```python
from build123d import *

# Parameters (mm, degrees)
SKETCH2_W           = 130
SKETCH2_H           = 70
BOSS_EXTRUDE1_DEPTH = 100
SKETCH3_W           = 104
SKETCH3_H           = 74
CUT_EXTRUDE1_DEPTH  = 67
SKETCH4_W           = 10
SKETCH4_H           = 10
CUT_EXTRUDE2_DEPTH  = 55
SKETCH5_W           = 104
SKETCH5_H           = 10
CUT_EXTRUDE3_DEPTH  = 67
SKETCH6_W           = 10
SKETCH6_H           = 74
CUT_EXTRUDE4_DEPTH  = 67
SKETCH9_R           = 1.75
CUT_EXTRUDE5_DEPTH  = 67
SKETCH10_R          = 4
CUT_EXTRUDE6_DEPTH  = 5
SKETCH12_R          = 4
CUT_EXTRUDE7_DEPTH  = 5
SKETCH13_R          = 4
CUT_EXTRUDE8_DEPTH  = 5
SKETCH14_R          = 4
CUT_EXTRUDE9_DEPTH  = 5
SKETCH15_W          = 3
SKETCH15_H          = 3
BOSS_EXTRUDE2_DEPTH = 5


with BuildPart() as part:
    # Sketch2 → Boss-Extrude1 (new body)
    with BuildSketch(Plane(origin=(0, 0, 0), x_dir=(1, 0, 0), z_dir=(0, 1, 0))):
        with Locations((65, 35)):
            Rectangle(SKETCH2_W, SKETCH2_H)
    extrude(amount=BOSS_EXTRUDE1_DEPTH)

    # Sketch3 → Cut-Extrude1 (cut)
    with BuildSketch(Plane(origin=(0, 0, -70), x_dir=(-1, 0, 0), z_dir=(0, 0, -1))):
        with Locations((-65, 50)):
            Rectangle(SKETCH3_W, SKETCH3_H)
    extrude(amount=-CUT_EXTRUDE1_DEPTH, mode=Mode.SUBTRACT)

    # Sketch4 → Cut-Extrude2 (cut)
    with BuildSketch(Plane.XY):
        with Locations((5, 95)):
            Rectangle(SKETCH4_W, SKETCH4_H)
        with Locations((125, 95)):
            Rectangle(SKETCH4_W, SKETCH4_H)
        with Locations((5, 5)):
            Rectangle(SKETCH4_W, SKETCH4_H)
        with Locations((125, 5)):
            Rectangle(SKETCH4_W, SKETCH4_H)
    extrude(amount=-CUT_EXTRUDE2_DEPTH, mode=Mode.SUBTRACT)

    # Sketch5 → Cut-Extrude3 (cut)
    with BuildSketch(Plane(origin=(0, 0, -70), x_dir=(-1, 0, 0), z_dir=(0, 0, -1))):
        with Locations((-65, 92)):
            Rectangle(SKETCH5_W, SKETCH5_H)
        with Locations((-65, 8)):
            Rectangle(SKETCH5_W, SKETCH5_H)
    extrude(amount=-CUT_EXTRUDE3_DEPTH, mode=Mode.SUBTRACT)

    # Sketch6 → Cut-Extrude4 (cut)
    with BuildSketch(Plane(origin=(0, 0, -70), x_dir=(-1, 0, 0), z_dir=(0, 0, -1))):
        with Locations((-122, 50)):
            Rectangle(SKETCH6_W, SKETCH6_H)
        with Locations((-8, 50)):
            Rectangle(SKETCH6_W, SKETCH6_H)
    extrude(amount=-CUT_EXTRUDE4_DEPTH, mode=Mode.SUBTRACT)

    # Sketch9 → Cut-Extrude5 (cut)
    with BuildSketch(Plane(origin=(0, 0, -70), x_dir=(-1, 0, 0), z_dir=(0, 0, -1))):
        with Locations((-124, 94)):
            Circle(SKETCH9_R)
        with Locations((-124, 6)):
            Circle(SKETCH9_R)
        with Locations((-6, 94)):
            Circle(SKETCH9_R)
        with Locations((-6, 6)):
            Circle(SKETCH9_R)
    extrude(amount=-CUT_EXTRUDE5_DEPTH, mode=Mode.SUBTRACT)

    # Sketch10 → Cut-Extrude6 (cut)
    with BuildSketch(Plane.XY.offset(-55)):
        with Locations((124, 94)):
            Circle(SKETCH10_R)
    extrude(amount=-CUT_EXTRUDE6_DEPTH, mode=Mode.SUBTRACT)

    # Sketch12 → Cut-Extrude7 (cut)
    with BuildSketch(Plane.XY.offset(-55)):
        with Locations((124, 6)):
            Circle(SKETCH12_R)
    extrude(amount=-CUT_EXTRUDE7_DEPTH, mode=Mode.SUBTRACT)

    # Sketch13 → Cut-Extrude8 (cut)
    with BuildSketch(Plane.XY.offset(-55)):
        with Locations((6, 6)):
            Circle(SKETCH13_R)
    extrude(amount=-CUT_EXTRUDE8_DEPTH, mode=Mode.SUBTRACT)

    # Sketch14 → Cut-Extrude9 (cut)
    with BuildSketch(Plane.XY.offset(-55)):
        with Locations((6, 94)):
            Circle(SKETCH14_R)
    extrude(amount=-CUT_EXTRUDE9_DEPTH, mode=Mode.SUBTRACT)

    # Sketch15 → Boss-Extrude2 (add)
    with BuildSketch(Plane(origin=(0, 0, -70), x_dir=(-1, 0, 0), z_dir=(0, 0, -1))):
        with Locations((-118.5, 88.5)):
            Rectangle(SKETCH15_W, SKETCH15_H)
        with Locations((-118.5, 11.5)):
            Rectangle(SKETCH15_W, SKETCH15_H)
        with Locations((-11.5, 11.5)):
            Rectangle(SKETCH15_W, SKETCH15_H)
        with Locations((-11.5, 88.5)):
            Rectangle(SKETCH15_W, SKETCH15_H)
    extrude(amount=BOSS_EXTRUDE2_DEPTH)


solid = part.part
```
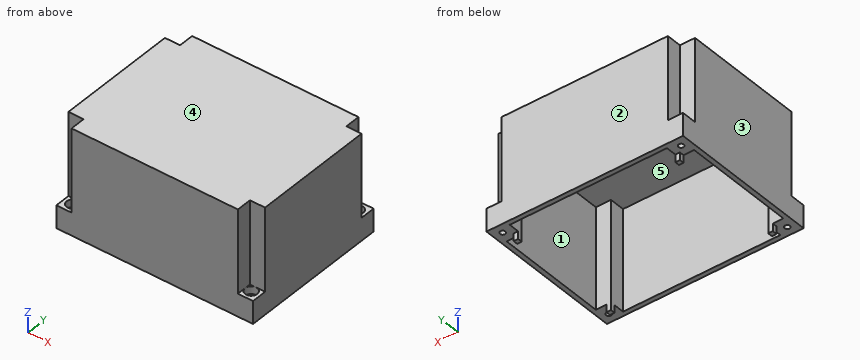
Geometry: final body of the model. Coordinates: model frame, mm. Face numbers are marked on the shaded views. A direction names the side the tool comes from. Round coordinates to 2 decimals unless told otherwise and drop trailing zeros. Write each loop counter-clockwise with the first axis right and the second up, starting at its lowest first coordinate (ties: lowest second). Pieces come first, ordered by that corner, then holes. Notation, with made-up numbers: M 6,43.5 L 18,43.5 A26 cw 18,77.5 Z; hole C 61.25,13.5 d5. An arc over 180 degrees is marked long. Answer in a Markdown table with one row per item. Add a question column.
(1) Draft query along X for the marked faces 3, 4 and 5. Return one class per face: pulls with the +X half, pulls with the -X half, needs draft (parallel to the pull), parting line crosses it, or undercut.
(2) Ray query, L1, parallel to X at y = 94, z = -57; L2, parallel to Y at x = 6, z = -57; L3, parallel to X at y = 94, z = -65.25. Return the intervals inside material, ascending.
(3) Cut plane C-C, the plane z = -30.5. Return the cut outline in (x, y).
(4) Reachability of the marked faces 1 and 2 from +Z, -Z, +X, -X, +Y, -Y: full face, straight path, thin tool, end or side. Return the list, or none.
(5) Contact query for flat-ended pins moving along their axis: pin 1 (1.5 mm diameter, centred on x = 86.5, y = 69, fed in from -Z); pin 2 (2.5 mm diameter, centred on y = 89, z = -73, fed in from +X); pin 3 (3 mm diameter, centred on x = 5.5, z = -14.5, fed in from +Y). Output: stop coordinate, or through.
(6) Cut plane D-D, the plane y = 16.5. Return the cut outline in (x, z), then the cut area to 3 significant figures.
(7) Cut plane B-B, the plane x = 72.5. Return the cut outline in (y, z).
(8) Cut plane A-A, the plane z = -66.5. Return the cut outline in (x, y).
Established:
| question | item | result |
|---|---|---|
| 1 | face 3 | pulls with the -X half |
| 1 | face 4 | needs draft |
| 1 | face 5 | undercut |
| 2 | L1 | 0 to 2, 10 to 13, 117 to 120, 128 to 130 |
| 2 | L2 | 0 to 2, 10 to 13, 87 to 90, 98 to 100 |
| 2 | L3 | 0 to 4.25, 7.75 to 13, 117 to 122.25, 125.75 to 130 |
| 3 | outline | M 0,10 L 10,10 L 10,0 L 120,0 L 120,10 L 130,10 L 130,90 L 120,90 L 120,100 L 10,100 L 10,90 L 0,90 Z; hole M 3,13 L 13,13 L 13,3 L 117,3 L 117,13 L 127,13 L 127,87 L 117,87 L 117,97 L 13,97 L 13,87 L 3,87 Z |
| 4 | face 1 | -Z |
| 4 | face 2 | +Z, -Z, +X, -X, +Y |
| 5 | pin 1 | z = -3 |
| 5 | pin 2 | x = 120 |
| 5 | pin 3 | y = 90 |
| 6 | outline | M 0,-70 L 3,-70 L 3,-3 L 127,-3 L 127,-70 L 130,-70 L 130,0 L 0,0 Z |
| 6 | area | 792 mm² |
| 7 | outline | M 0,-70 L 3,-70 L 3,-3 L 97,-3 L 97,-70 L 100,-70 L 100,0 L 0,0 Z |
| 8 | outline | M 0,0 L 130,0 L 130,100 L 0,100 Z; hole M 3,13 L 13,13 L 13,3 L 117,3 L 117,13 L 127,13 L 127,87 L 117,87 L 117,97 L 13,97 L 13,87 L 3,87 Z; hole C 6,6 d3.5; hole C 6,94 d3.5; hole C 124,6 d3.5; hole C 124,94 d3.5 |
